```python
from build123d import *

# Parameters (mm, degrees)
CHANFRO1_SIZE               = 1
FURO_COM_FOLGA_DE_M61_D     = 6.6
FURO_COM_FOLGA_DE_M61_DEPTH = 23.799
FURO_COM_FOLGA_DE_M61_TIP   = 1.982840043


with BuildPart() as part:
    # Esboço1 → Revolução1 (revolve)
    with BuildSketch(Plane.XY):
        with BuildLine():
            Line((96.4, 0), (96.4, 13.8))
            Line((96.4, 13.8), (52, 13.8))
            ThreePointArc((52, 13.8), (50.585786438, 14.385786438), (50, 15.8))
            Line((50, 15.8), (50, 44.8))
            Line((50, 44.8), (38.1, 44.8))
            Line((38.1, 44.8), (38.1, 0))
            Line((38.1, 0), (96.4, 0))
        make_face()
    revolve(axis=Axis((0, 0, 0), (0, 1, 0)))

    # Chanfro1
    chanfro1_edges = [part.edges().sort_by_distance(p)[0] for p in [
        (-96.4, 0, 0),
        (-96.4, 13.8, 0),
        (-50, 44.8, 0),
        (-38.1, 0, 0),
    ]]
    chamfer(chanfro1_edges, length=CHANFRO1_SIZE)

    # Furo com folga de M61
    with Locations(Plane.ZX.offset(13.8)):
        with Locations((0, 73.7), (73.7, 0), (0, -73.7), (-73.7, 0), (0, 0)):
            Hole(FURO_COM_FOLGA_DE_M61_D / 2, depth=FURO_COM_FOLGA_DE_M61_DEPTH)
            with Locations((0, 0, -(FURO_COM_FOLGA_DE_M61_DEPTH + FURO_COM_FOLGA_DE_M61_TIP / 2))):  # 118° drill point
                Cone(0, FURO_COM_FOLGA_DE_M61_D / 2, FURO_COM_FOLGA_DE_M61_TIP, mode=Mode.SUBTRACT)


solid = part.part
```
The model under review builds one solid part; all positions refer to its coordinate system, in mm. A direction names the side the tool comes from. Round coordinates to 2 decimals unless told otherwise and drop trailing zeros. Answer in a Markdown table with one row per item.
(1) Machinability: for faces 1 (the face through (47.69, 30, -15.02)), 2 (the face through (-70.917, 6.803, -1.774)), which of the approach directions +Z, -Z, +X, -X, +Y, -Y give a long, thin tool a straight path to every point of the face, cutting with its end or side? Answer none if there is none.
Result set:
| item | result |
|---|---|
| face 1 | +Y |
| face 2 | +Y, -Y |
(2) Clearance check with flat-ended pins moving along their axes: P1, Ø12, axis at x = -57, y = 22, coming from the +Z side; P2, Ø6, axis at x = -60, y = 14.5, coming from the -Z side; P3, Ø10, axis at y = 20.5, z = 23.5, coming from the +X side; P4, Ø3, axis at y = 7, z = 30, coming from the +X side. State where each tip first meets the part, or that it passes through.
Result set:
| item | result |
|---|---|
| P1 | passes through |
| P2 | stops at z = -77.35 |
| P3 | stops at x = 46.45 |
| P4 | stops at x = 92.09 |
(3) Take a section at A-A on x = 0. Count the separate pieces of the cut face and the enclosed holes in it, plus the area to 3 significant figures.
Result set:
| item | result |
|---|---|
| separate pieces | 4 |
| enclosed holes | 0 |
| area | 2,160 mm2 |
(4) For line 1 (X direction, y = 9, z = 0); line 2 (Z direction, x = 0.5, y = 21.5); line 3 (Y direction, x = 39, z = 75.5), list the stretches that pass through material, from the lowest coordinate up. Write a range as from..to.
Result set:
| item | result |
|---|---|
| line 1 | x = -96.4..-77, -70.4..-38.1, 38.1..70.4, 77..96.4 |
| line 2 | z = -50..-38.1, 38.1..50 |
| line 3 | y = 0..13.8 |
(5) Mouldability with a two-part tool opening along X and no side actions: class faces 3 (the face through (-30.235, 22.593, 23.183)), 4 (the face through (-41, 0, -1)), 5 (the face through (-71.05, 6.98, -65.15)) as released by +X, released by -X, zero draft, split by the parting line, or undercut.
Result set:
| item | result |
|---|---|
| face 3 | undercut |
| face 4 | zero draft |
| face 5 | split by the parting line |
